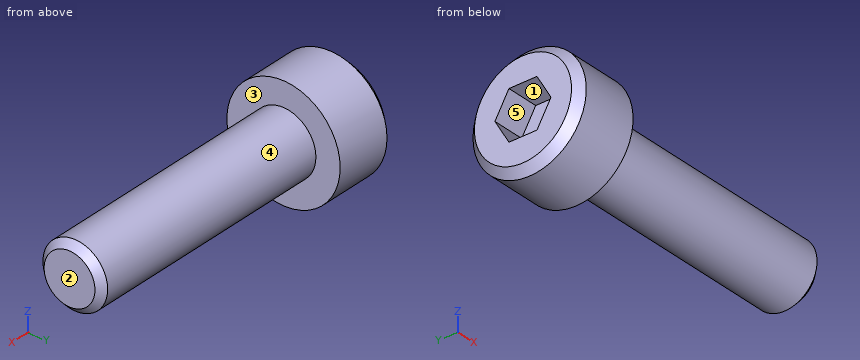
Autodesk Inventor part; units mm, degrees
ref_plane "PPBF_KEDS_XY" through (4, 0, 0) normal (-1, 0, 0) x (0, 0, -1)
ref_plane "PPBF_KEDS_YZ" through (4, 0, 0) normal (0, 0, -1) x (0, -1, 0)
ref_plane "PPBF_KEDS_ZX" through (4, 0, 0) normal (0, -1, 0) x (-1, 0, 0)
sketch "__1" plane through (0, 0, 0) normal (0, 0, 1) x (1, 0, 0)
  line L0 (66, 0) -> (-66, 0)
  line L1 (0, 0) -> (0, 3.5)
  line L2 (0, 3.5) -> (4, 3.5)
  line L3 (4, 3.5) -> (4, 2)
  line L4 (4, 2) -> (19.5705, 2)
  line L5 (19.5705, 2) -> (20, 1.5705)
  line L6 (20, 1.5705) -> (20, 0)
  line L7 (20, 0) -> (0, 0)
revolve "Revolution1" add sketch "__1" angle 360 about axis through (66, 0, 0) along (1, 0, 0)
thread "Thread1"
sketch "__2" plane through (0, 0, 0) normal (1, 0, 0) x (0, 0, -1)
  line L0 (-1.5, -0.866) -> (0, -1.7321)
  line L1 (0, -1.7321) -> (1.5, -0.866)
  line L2 (1.5, -0.866) -> (1.5, 0.866)
  line L3 (1.5, 0.866) -> (0, 1.7321)
  line L4 (0, 1.7321) -> (-1.5, 0.866)
  line L5 (-1.5, 0.866) -> (-1.5, -0.866)
extrude "Extrusion1" cut sketch "__2" along normal blind 2
chamfer "Chamfer1" distance 0.5 angle 45 1 edges at (0, -3.5, 0)
ref_plane "PPBF_KEDS_XY" through (4, 0, 0) normal (-1, 0, 0) x (0, 0, -1)
ref_plane "PPBF_KEDS_YZ" through (4, 0, 0) normal (0, 0, -1) x (0, -1, 0)
ref_plane "PPBF_KEDS_ZX" through (4, 0, 0) normal (0, -1, 0) x (-1, 0, 0)
properties part number "CBB4-16"
Could you check a few things on this model? Use its own coordinates, in mm. Face numbers are marked on the shaded views. A direction names the side the tool comes from. Give positions to 0.01 mm unless a question says otherwise; leave off trailing zeros. Order: outer loops, then holes, each group sorted by start corner. A loop starts at its lowest first (then second) coordinate and runs counter-clockwise, first axis right, second up.
1. Suppose I cut it at B-B (y = 0). Write out the boundary of the cut face in (x, z).
Answers below:
outline: (0, -3) - (0.5, -3.5) - (4, -3.5) - (4, -2) - (19.57, -2) - (20, -1.57) - (20, 1.57) - (19.57, 2) - (4, 2) - (4, 3.5) - (0.5, 3.5) - (0, 3) - (0, 1.5) - (2, 1.5) - (2, -1.5) - (0, -1.5) - close
2. Thinking about a two-plate mould opening in Y: for the marked faces 3, 4 and 5, which applies, +Y half, -Y half, draft (parallel to the pull), parting line (faces both ways), or undercut?
Answers below:
face 3: draft
face 4: parting line
face 5: undercut
3. Which directions (+Z, -Z, +X, -X, +Y, -Y) give clear straight access to the entire face, cutting with the end or side of a thin tool? Please do the marked faces 1 and 2.
Answers below:
face 1: -X
face 2: +Z, -Z, +X, +Y, -Y
4. I need wall thicknesses on L1, parallel to X at y = -0.5, z = -2.75; L2, parallel to Z at x = 16.5, y = 0; L3, parallel to X at y = 0.25, z = -0.5. Which ranges of each line are inside material? Lowest first, please.
Answers below:
L1: x = 0 to 4
L2: z = -2 to 2
L3: x = 2 to 20
5. For pin 1 (2 mm diameter, centred on x = 3.5, z = 1.5, fed in from +Y); pin 2 (2 mm diameter, centred on x = 12.5, z = -2, fed in from -Y); pin 3 (4 mm diameter, centred on x = 7, y = 0.5, fed in from +Z), each with a flat end and sliding along its axis, tell me the tip position at first contact or that it passes through.
Answers below:
pin 1: stops at y = 3.46
pin 2: stops at y = -1.73
pin 3: stops at z = 2
6. Suppose I cut it at A-A (x = 1.75). Write out the boundary of the cut face in (y, z), plus the area to 3 significant figures.
Answers below:
outline: circle Ø7 at (0, 0); hole (-1.73, 0) - (-0.87, -1.5) - (0.87, -1.5) - (1.73, 0) - (0.87, 1.5) - (-0.87, 1.5) - close
area: 30.7 mm2
7. Suppose I cut it at C-C (x = 10.5). Write out the boundary of the cut face in (y, z), plus the area to 3 significant figures.
Answers below:
outline: circle Ø4 at (0, 0)
area: 12.6 mm2
